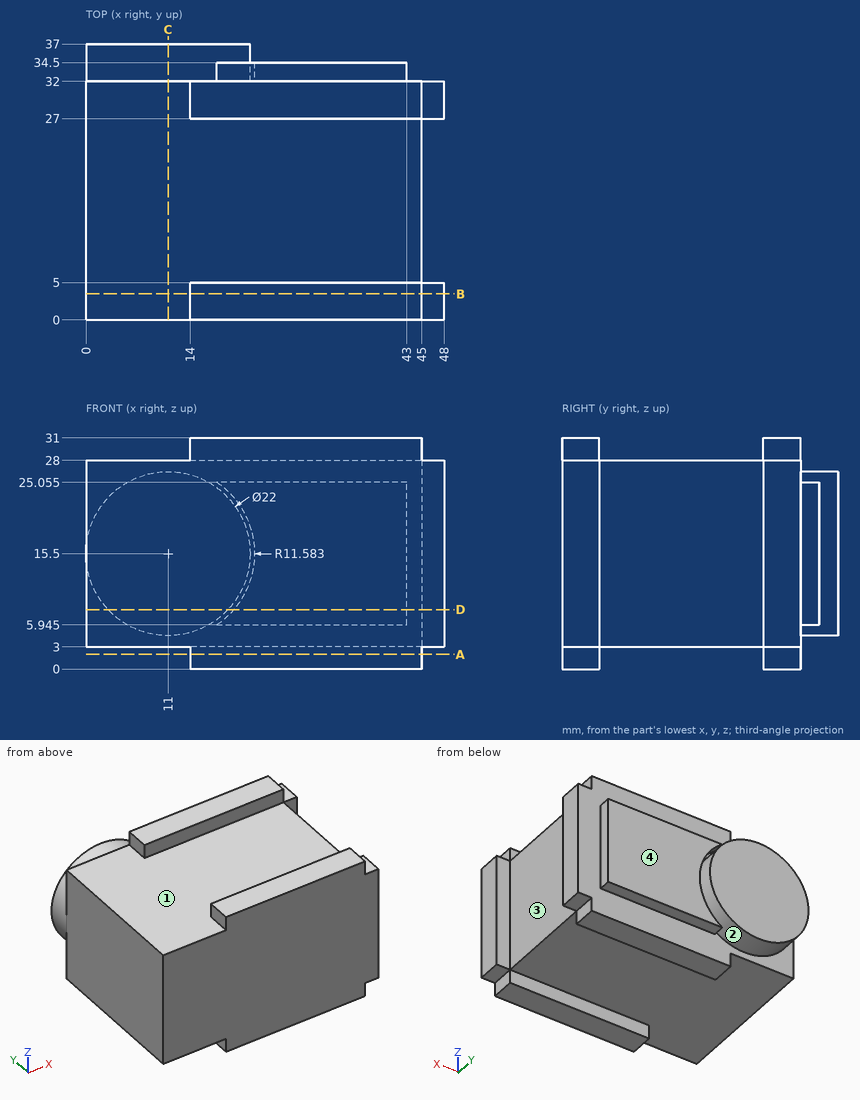
The drawing under review shows one solid part. Ordinate dimensions are in mm from its lowest x, y, z. Coordinates: 2 decimals unless noted, no trailing zeros. Write each loop counter-clockwise with the first axis right and the second up, starting at its lowest first coordinate (ties: lowest second). Pieces come first, ordered by that corner, then holes. Notation, with made-up numbers: (52, 27) - (106, 27) arc R27 cw to (106, 49) - close; hole circle Ø9 at (42, 66.25). An arc over 180 degrees is marked (long way). Answer as CSV lines item,"result".
(1) For line 1 along Z through (x, y) = (6.5, 14); line 2 along Y through (x, z) = (41.5, 21); line 3 along X through (y, z) = (17, 15.5), list the stretches that pass through material, from the lowest coordinate up. Write a range as [from, to].
Data:
line 1,"z = [3, 28]"
line 2,"y = [0, 34.5]"
line 3,"x = [0, 45]"
(2) Clearance check with flat-ended pins moving along their axes: pin 1 Ø1.2 at (x, y) = (26, 33.5) entering from -Z (3 decimals); pin 2 Ø1.5 at (x, z) = (27, 27) entering from +Y; pin 3 Ø3.5 at (x, y) = (47, 3.5) entering from +Z. State where each tip first meets the part, or that it passes through.
Data:
pin 1,"stops at z = 5.945"
pin 2,"stops at y = 32"
pin 3,"stops at z = 28"
(3) We need section A-A (z = 2). Give the boundary of the cut face in (x, y), plus the area to 3 significant figures.
Data:
outline,"(14, 0) - (45, 0) - (45, 5) - (14, 5) - close; (14, 27) - (45, 27) - (45, 32) - (14, 32) - close"
area,"310 mm2"
(4) We need section B-B (y = 3.5). Give the boundary of the cut face in (x, z), plus the area to 3 significant figures.
Data:
outline,"(0, 3) - (14, 3) - (14, 0) - (45, 0) - (45, 3) - (48, 3) - (48, 28) - (45, 28) - (45, 31) - (14, 31) - (14, 28) - (0, 28) - close"
area,"1,390 mm2"
(5) We need section C-C (x = 11). Give the boundary of the cut face in (y, z).
Data:
outline,"(0, 3) - (32, 3) - (32, 4.5) - (37, 4.5) - (37, 26.5) - (32, 26.5) - (32, 28) - (0, 28) - close"
(6) We need section D-D (z = 8). Give the boundary of the cut face in (x, y), plus the area to 3 significant figures.
Data:
outline,"(0, 0) - (48, 0) - (48, 5) - (45, 5) - (45, 27) - (48, 27) - (48, 32) - (43, 32) - (43, 34.5) - (19.83, 34.5) - (19.83, 32) - (19.05, 32) - (19.05, 37) - (2.95, 37) - (2.95, 32) - (0, 32) - close"
area,"1,610 mm2"
(7) Mouldability with a two-part tool opening along Y and no side actions: class the marked faces 1, 2, 3 and 4 as pulls with the +Y half, pulls with the -Y half, needs draft (parallel to the pull), parting line crosses it, or undercut.
Data:
face 1,"undercut"
face 2,"needs draft"
face 3,"undercut"
face 4,"pulls with the +Y half"
